```python
from build123d import *

# Parameters (mm, degrees)
F0_W     = 101.6
F0_H     = 59.0938783061
F1_DEPTH = 127
F2_T     = -2.54
F4_W     = 59.033177793
F4_H     = 79.0090560913
F5_DEPTH = 2.54


with BuildPart() as f1:
    # F0 (on Top) → F1 (new body)
    with BuildSketch(Plane.XY):
        with Locations((-1.5831552446, -2.7139894664)):
            Rectangle(F0_W, F0_H)
    extrude(amount=F1_DEPTH)

    # F2
    f2_openings = [f1.faces().sort_by_distance(p)[0] for p in [
        (49.216845, -2.713989, 63.5),
    ]]
    offset(amount=F2_T, openings=f2_openings)

    # F4 (on offset) → F5 (join)
    with BuildSketch(Plane.YZ.offset(49.2168447554)):
        with Locations((-2.5649182498, 87.9480838776)):
            Rectangle(F4_W, F4_H)
    extrude(amount=-F5_DEPTH)


solid = f1.part
```
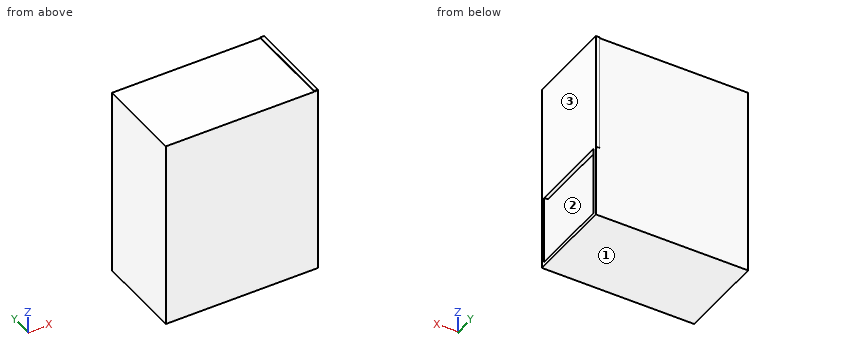
Can you work these out from the model? Positions are in its coordinate system, mm. Face numbers are marked on the shaded views. Round coordinates to 2 decimals unless told otherwise and drop trailing zeros. Loops run counter-clockwise (first coordinate to the right, second up) from the corner with the lowest first, then second, coordinate; pieces in that order, holes last. Notation, with made-up numbers: M 64,62.5 L 90,62.5 A26 ccw 90,99.5 Z; hole C 68,18.5 d11. An arc over 180 degrees is marked long. Answer as a JSON object with one key per item and string values. Group by question number.
Q1. Imagine slicing it at C-C, the plane y = -9.5. Please give me the cut outline in (x, z), then the cut area to 3 significant figures.
Q2. Imagine slicing it at B-B, the plane z = 59. Please give me the cut outline in (x, y), then the cut area to 3 significant figures.
Q3. Please list where these lines run through material, in increasing order: L1, parallel to Y at x = 20, z = 98; L2, parallel to X at y = 6.5, z = 113; L3, parallel to Z at x = -46.5, y = 13.5.
Q4. Will these pins go through, and if not, where does the flat tip stop? pin 1 (3 mm diameter, centred on x = 17.5, y = -1.5, fed in from +Z); pin 2 (2 mm diameter, centred on x = 48.5, y = -9.5, fed in from -Z); pin 3 (1.5 mm diameter, centred on y = 19.5, z = 19.5, fed in from +X); pin 4 (10 mm diameter, centred on x = 27.5, z = 50.5, fed in from +Y).
Q5. Imagine slicing it at A-A, the plane x = -11. Please give me the cut outline in (y, z).
Q6. We'd pull the mould along Z, two halves only. Please class the marked faces 1, 2 and 3: +Z half, -Z half, draft (parallel to the pull), parting line (faces both ways), or undercut.
Findings:
{
 "1": {"outline": "M -52.38,0 L 49.22,0 L 49.22,2.54 L -49.84,2.54 L -49.84,124.46 L 46.68,124.46 L 46.68,48.44 L 49.22,48.44 L 49.22,127.45 L 46.68,127.45 L 46.68,127 L -52.38,127 Z", "area": "1,020 mm2"},
 "2": {"outline": "M -52.38,-32.26 L 49.22,-32.26 L 49.22,26.95 L 46.68,26.95 L 46.68,26.83 L -52.38,26.83 Z; hole M -49.84,-29.72 L 46.68,-29.72 L 46.68,24.29 L -49.84,24.29 Z", "area": "791 mm2"},
 "3": {"L1": "y = -32.26 to -29.72, 24.29 to 26.83", "L2": "x = -52.38 to -49.84, 46.68 to 49.22", "L3": "z = 0 to 2.54, 124.46 to 127"},
 "4": {"pin 1": "stops at z = 127", "pin 2": "stops at z = 0", "pin 3": "stops at x = -49.84", "pin 4": "stops at y = 26.83"},
 "5": {"outline": "M -32.26,0 L 26.83,0 L 26.83,127 L -32.26,127 Z; hole M -29.72,2.54 L 24.29,2.54 L 24.29,124.46 L -29.72,124.46 Z"},
 "6": {"face 1": "-Z half", "face 2": "undercut", "face 3": "draft"}
}
